from build123d import *

# Parameters (mm, degrees)
SKETCH014_R         = 1.6
PAD004_DEPTH        = 3
POCKET011_DEPTH     = 3.00101
LINEARPATTERN_COUNT = 2
LINEARPATTERN_PITCH = 50


with BuildPart() as part:
    # Sketch014 (on Binder) → Pad004 (new body)
    with BuildSketch(Plane(origin=(1.2e-05, -70, 0), x_dir=(1, 0, 0), z_dir=(0, -1, 0))):
        with BuildLine():
            ThreePointArc((-26.75, 111), (-28.87132, 110.12132), (-29.75, 108))
            Line((-29.75, 14), (-29.75, 108))
            ThreePointArc((-29.75, 14), (-28.87132, 11.87868), (-26.75, 11))
            Line((26.75, 11), (-26.75, 11))
            ThreePointArc((26.75, 11), (28.87132, 11.87868), (29.75, 14))
            Line((29.75, 108), (29.75, 14))
            ThreePointArc((29.75, 108), (28.87132, 110.12132), (26.75, 111))
            Line((-26.75, 111), (26.75, 111))
        make_face()
        with Locations((-25.75, 97)):
            Circle(SKETCH014_R, mode=Mode.SUBTRACT)
        with Locations((25.75, 97)):
            Circle(SKETCH014_R, mode=Mode.SUBTRACT)
        with Locations((25.75, 56)):
            Circle(SKETCH014_R, mode=Mode.SUBTRACT)
        with Locations((-25.75, 56)):
            Circle(SKETCH014_R, mode=Mode.SUBTRACT)
        with Locations((-25.75, 15)):
            Circle(SKETCH014_R, mode=Mode.SUBTRACT)
        with Locations((25.75, 15)):
            Circle(SKETCH014_R, mode=Mode.SUBTRACT)
        with Locations((-25.75, 106.751)):
            Circle(SKETCH014_R, mode=Mode.SUBTRACT)
        with Locations((25.75, 106.751)):
            Circle(SKETCH014_R, mode=Mode.SUBTRACT)
    extrude(amount=PAD004_DEPTH)

    # Sketch019 (on Face18 of Pad004) → Pocket011 (cut, through all)
    with BuildSketch(Plane(origin=(1.2e-05, -73, 0), x_dir=(1, 0, 0), z_dir=(0, -1, 0))):
        with BuildLine():
            ThreePointArc((-6, 86), (-7.5, 87.5), (-9, 86))
            Line((-9, 86), (-9, 76))
            ThreePointArc((-9, 76), (-7.5, 74.5), (-6, 76))
            Line((-6, 76), (-6, 86))
        make_face()
        with BuildLine():
            ThreePointArc((9, 86), (7.5, 87.5), (6, 86))
            Line((6, 86), (6, 76))
            ThreePointArc((6, 76), (7.5, 74.5), (9, 76))
            Line((9, 76), (9, 86))
        make_face()
    pocket011 = extrude(amount=-POCKET011_DEPTH, mode=Mode.SUBTRACT)

    # LinearPattern: Pocket011 ×2
    with Locations(*[(0, 0, -i * LINEARPATTERN_PITCH) for i in range(1, LINEARPATTERN_COUNT)]):
        add(pocket011, mode=Mode.SUBTRACT)


solid = part.part
For this review, take the finished solid that the model builds, in its own axes (mm). A direction names the side the tool comes from. Coordinates: 2 decimals unless noted, no trailing zeros. Write each loop counter-clockwise with the first axis right and the second up, starting at its lowest first coordinate (ties: lowest second). Pieces come first, ordered by that corner, then holes. Notation, with made-up numbers: (-36, 39.25) -> (3, 39.25) arc R18 ccw to (3, 67.25) -> close; hole circle Ø7 at (-10, 12.25). An arc over 180 degrees is marked (long way). Write each question's results on one line, items separated by ' | '. Start each with the question number.
1) Insertion check: pin 1 (1.9 mm diameter, centred on x = -25.75, z = 56, fed in from +Y). The pin has a flat end and moves straight along its axis. Give the tip position at first contact, or say it passes through.
2) Consider section C-C (z = 83). Write out the cut boundary in (x, y), plus the area to 4 significant figures.
3) Wall thickness on L1, parallel to X at y = -72.5, z = 27; L2, parallel to Z at x = -26, y = -71.2; L3, parallel to Z at x = 8, y = -70.35: over which ranges is each line inside the solid? List them lowest first. Write a range as [from, to].
4) The part is to be moulded in two halves that separate along Z. For faces 1 (the face through (-28.89, -71.48, 11.9)), 2 (the face through (7.5, -71.5, 24.5)), 3 (the face through (0, -71, 111)), 4 (the face through (-29.75, -71, 60)), say which applies: +Z half, -Z half, draft (parallel to the pull), parting line (faces both ways), or undercut.
5) Consider section B-B (y = -72.3). Give the number of separate pieces and of enclosed holes in the cut face, plus the area to 3 significant figures.
6) For faces 5 (the face through (-28.85, -71.48, 110.14)), 6 (the face through (6, -72, 31)), list the 3-axis set-ups (+Z, -Z, +X, -X, +Y, -Y) from which the entire face can be reached by the end or side of a thin tool; tool diameter is ignored.
7) Consider section A-A (z = 97). Write out the cut boundary in (x, y), plus the area to 3 significant figures.
Geometry says:
1) pin 1: through
2) outline: (-29.75, -73) -> (-9, -73) -> (-9, -70) -> (-29.75, -70) -> close; (-6, -73) -> (6, -73) -> (6, -70) -> (-6, -70) -> close; (9, -73) -> (29.75, -73) -> (29.75, -70) -> (9, -70) -> close | area: 160.5 mm^2
3) L1: [-29.75, -9], [-6, 6], [9, 29.75] | L2: [11, 13.42], [16.58, 54.42], [57.58, 95.42], [98.58, 105.17], [108.33, 111] | L3: [11, 24.59], [37.41, 74.59], [87.41, 111]
4) face 1: -Z half | face 2: undercut | face 3: +Z half | face 4: draft
5) separate pieces: 1 | enclosed holes: 12 | area: 5,730 mm^2
6) face 5: +Z, -X, +Y, -Y | face 6: +Y, -Y
7) outline: (-29.75, -73) -> (-27.35, -73) -> (-27.35, -70) -> (-29.75, -70) -> close; (-24.15, -73) -> (24.15, -73) -> (24.15, -70) -> (-24.15, -70) -> close; (27.35, -73) -> (29.75, -73) -> (29.75, -70) -> (27.35, -70) -> close | area: 159 mm^2
